from build123d import *

# Parameters (mm, degrees)
F1_DEPTH = 1.5875
F2_DEPTH = 7.9375


with BuildPart() as f1:
    # F0 (on Top) → F1 (new body)
    with BuildSketch(Plane.XY):
        with BuildLine():
            ThreePointArc((-44.45, 0), (-31.4308964237, -31.4308964237), (0, -44.45))
            Line((0, -44.45), (0, -31.75))
            ThreePointArc((0, -31.75), (-21.3000274256, -23.5450914559), (-31.59125, -3.1710287664))
            ThreePointArc((-31.59125, -3.1710287664), (-33.9382177394, -2.3005060585), (-34.925, 0))
            Line((-34.925, 0), (-44.45, 0))
        make_face()
        with BuildLine():
            ThreePointArc((-31.59125, -3.1710287664), (-21.3000274256, -23.5450914559), (0, -31.75))
            Line((0, -31.75), (0, 0))
            Line((0, 0), (-28.575, 0))
            ThreePointArc((-28.575, 0), (-29.4494939415, -2.1882177394), (-31.59125, -3.1710287664))
        make_face()
        with BuildLine():
            Line((0, 0), (0, -31.75))
            ThreePointArc((0, -31.75), (21.3000274256, -23.5450914559), (31.59125, -3.1710287664))
            ThreePointArc((31.59125, -3.1710287664), (29.4494939415, -2.1882177394), (28.575, 0))
            Line((28.575, 0), (0, 0))
        make_face()
        with BuildLine():
            ThreePointArc((0, -44.45), (31.4308964237, -31.4308964237), (44.45, 0))
            Line((44.45, 0), (34.925, 0))
            ThreePointArc((34.925, 0), (33.9382177394, -2.3005060585), (31.59125, -3.1710287664))
            ThreePointArc((31.59125, -3.1710287664), (21.3000274256, -23.5450914559), (0, -31.75))
            Line((0, -31.75), (0, -44.45))
        make_face()
        with BuildLine():
            Line((34.925, 0), (44.45, 0))
            ThreePointArc((44.45, 0), (31.4308964237, 31.4308964237), (0, 44.45))
            Line((0, 44.45), (0, 31.75))
            ThreePointArc((0, 31.75), (21.3000274256, 23.5450914559), (31.59125, 3.1710287664))
            ThreePointArc((31.59125, 3.1710287664), (33.9382177394, 2.3005060585), (34.925, 0))
        make_face()
        with BuildLine():
            ThreePointArc((31.59125, 3.1710287664), (21.3000274256, 23.5450914559), (0, 31.75))
            Line((0, 31.75), (0, 0))
            Line((0, 0), (28.575, 0))
            ThreePointArc((28.575, 0), (29.4494939415, 2.1882177394), (31.59125, 3.1710287664))
        make_face()
        with BuildLine():
            Line((0, 0), (0, 31.75))
            ThreePointArc((0, 31.75), (-21.3000274256, 23.5450914559), (-31.59125, 3.1710287664))
            ThreePointArc((-31.59125, 3.1710287664), (-29.4494939415, 2.1882177394), (-28.575, 0))
            Line((-28.575, 0), (0, 0))
        make_face()
        with BuildLine():
            Line((0, 31.75), (0, 44.45))
            ThreePointArc((0, 44.45), (-31.4308964237, 31.4308964237), (-44.45, 0))
            Line((-44.45, 0), (-34.925, 0))
            ThreePointArc((-34.925, 0), (-33.9382177394, 2.3005060585), (-31.59125, 3.1710287664))
            ThreePointArc((-31.59125, 3.1710287664), (-21.3000274256, 23.5450914559), (0, 31.75))
        make_face()
    extrude(amount=F1_DEPTH)

    # F0 (on Top) → F2 (join)
    with BuildSketch(Plane.XY):
        with BuildLine():
            ThreePointArc((-31.59125, 3.1710287664), (-33.9382177394, 2.3005060585), (-34.925, 0))
            ThreePointArc((-34.925, 0), (-33.9382177394, -2.3005060585), (-31.59125, -3.1710287664))
            ThreePointArc((-31.59125, -3.1710287664), (-29.4494939415, -2.1882177394), (-28.575, 0))
            ThreePointArc((-28.575, 0), (-29.4494939415, 2.1882177394), (-31.59125, 3.1710287664))
        make_face()
        with BuildLine():
            ThreePointArc((31.59125, -3.1710287664), (33.9382177394, -2.3005060585), (34.925, 0))
            ThreePointArc((34.925, 0), (33.9382177394, 2.3005060585), (31.59125, 3.1710287664))
            ThreePointArc((31.59125, 3.1710287664), (29.4494939415, 2.1882177394), (28.575, 0))
            ThreePointArc((28.575, 0), (29.4494939415, -2.1882177394), (31.59125, -3.1710287664))
        make_face()
    extrude(amount=F2_DEPTH)


solid = f1.part
Can you work these out from the model? Positions are in its coordinate system, mm. Give positions to 0.01 mm unless a question says otherwise; leave off trailing zeros. Write each loop counter-clockwise with the first axis right and the second up, starting at its lowest first coordinate (ties: lowest second). Pieces come first, ordered by that corner, then holes. Notation, with made-up numbers: M 70.25,35.25 L 108.25,35.25 A5 ccw 108.25,40.25 Z; hole C 16.25,13.5 d9. An arc over 180 degrees is marked long. Answer in a Markdown table with one row per item. Add a question column.
Item 1: Imagine slicing it at C-C, the plane y = -28.5. Write out the boundary of the cut face in (x, z), plus the area to 3 significant figures.
Item 2: Please list where these lines run through material, in increasing order: L1, parallel to Z at x = -10, y = 4; L2, parallel to X at y = -1, z = 3; L3, parallel to Y at x = 24.5, z = 1.25.
Item 3: Imagine slicing it at B-B, the plane x = -20.5. Write out the boundary of the cut face in (y, z).
Item 4: For pin 1 Ø12 at (x, y) = (31.5, 14.5) entering from +Z; pin 2 Ø4 at (y, z) = (-19.5, 4.5) entering from -X; pin 3 Ø4 at (y, z) = (26.5, 2.5) entering from -X, each with a flat end and sliding along its axis, tell me the tip position at first contact or that it passes through.
Item 5: Imagine slicing it at A-A, the plane z = 5. Write out the boundary of the cut face in (x, y) (3 decimals).
Evaluation:
| question | item | result |
|---|---|---|
| 1 | outline | M -34.11,0 L 34.11,0 L 34.11,1.59 L -34.11,1.59 Z |
| 1 | area | 108 mm² |
| 2 | L1 | z = 0 to 1.59 |
| 2 | L2 | x = -34.76 to -28.74, 28.74 to 34.76 |
| 2 | L3 | y = -37.09 to 37.09 |
| 3 | outline | M -39.44,0 L 39.44,0 L 39.44,1.59 L -39.44,1.59 Z |
| 4 | pin 1 | stops at z = 1.59 |
| 4 | pin 2 | passes through |
| 4 | pin 3 | stops at x = -36.94 |
| 5 | outline | C -31.75,0 d6.35; C 31.75,0 d6.35 |
